```python
from build123d import *

# Parameters (mm, degrees)
F0_W     = 6.35
F0_H     = 88.9
F1_DEPTH = 3
F0_H_2   = 6.35
F0_W_2   = 12.7
F0_W_3   = 76.2
F2_DEPTH = 25.4
F0_W_4   = 25.4
F3_DEPTH = 8


with BuildPart() as f1:
    # F0 (on Front) → F1 (new body)
    with BuildSketch(Plane.XZ):
        with Locations((-59.3524831653, 10.6868692262)):
            Rectangle(F0_W, F0_H)
        Polygon((-43.4774831653, 55.1368692262), (-56.1774831653, 55.1368692262), (-56.1774831653, -33.7631307738), (-43.4774831653, -33.7631307738), (-18.0774831653, -33.7631307738), (58.1225168347, -33.7631307738), (83.5225168347, -33.7631307738), (96.2225168347, -33.7631307738), (96.2225168347, 55.1368692262), (83.5225168347, 55.1368692262), (58.1225168347, 55.1368692262), (-18.0774831653, 55.1368692262), align=None)
    extrude(amount=F1_DEPTH)

    # F0 (on Front) → F2 (join)
    with BuildSketch(Plane.XZ):
        with Locations((-59.3524831653, 58.3118692262)):
            Rectangle(F0_W, F0_H_2)
        with Locations((99.3975168347, 58.3118692262)):
            Rectangle(F0_W, F0_H_2)
        with Locations((-59.3524831653, -36.9381307738)):
            Rectangle(F0_W, F0_H_2)
        with Locations((99.3975168347, -36.9381307738)):
            Rectangle(F0_W, F0_H_2)
        with Locations((-49.8274831653, 58.3118692262)):
            Rectangle(F0_W_2, F0_H_2)
        with Locations((20.0225168347, 58.3118692262)):
            Rectangle(F0_W_3, F0_H_2)
        with Locations((89.8725168347, 58.3118692262)):
            Rectangle(F0_W_2, F0_H_2)
        with Locations((-49.8274831653, -36.9381307738)):
            Rectangle(F0_W_2, F0_H_2)
        with Locations((20.0225168347, -36.9381307738)):
            Rectangle(F0_W_3, F0_H_2)
        with Locations((89.8725168347, -36.9381307738)):
            Rectangle(F0_W_2, F0_H_2)
        with Locations((99.3975168347, 10.6868692262)):
            Rectangle(F0_W, F0_H)
        with Locations((-59.3524831653, 10.6868692262)):
            Rectangle(F0_W, F0_H)
    extrude(amount=F2_DEPTH)

    # F0 (on Front) → F3 (join)
    with BuildSketch(Plane.XZ):
        with Locations((-30.7774831653, -36.9381307738)):
            Rectangle(F0_W_4, F0_H_2)
        with Locations((-30.7774831653, 58.3118692262)):
            Rectangle(F0_W_4, F0_H_2)
        with Locations((70.8225168347, 58.3118692262)):
            Rectangle(F0_W_4, F0_H_2)
        with Locations((70.8225168347, -36.9381307738)):
            Rectangle(F0_W_4, F0_H_2)
    extrude(amount=F3_DEPTH)


solid = f1.part
```
The listing builds one solid part. Answer for the finished solid, in the listing's coordinates (mm). A direction names the side the tool comes from. Give positions to 0.01 mm unless a question says otherwise; leave off trailing zeros. Loops run counter-clockwise (first coordinate to the right, second up) from the corner with the lowest first, then second, coordinate; pieces in that order, holes last. Notation, with made-up numbers: (24.5, -12) - (70.5, -12) arc R5 cw to (70.5, -4) - close; hole circle Ø11 at (-23.5, -29). An arc over 180 degrees is marked (long way). Answer as CSV lines item,"result". Start each with the question number.
Item 1: A cutting plane is placed at A-A on y = -9.75. Determine the outline of the cut face in (x, z).
Item 2: A cutting plane is placed at B-B on x = 15. Determine the outline of the cut face in (y, z), then the cut area to 3 significant figures.
Item 3: Each of these flat-tipped pins is pushed along its axis until it touches: pin 1 (12 mm diameter, centred on x = 67, z = 15.5, fed in from +Y); pin 2 (7 mm diameter, centred on x = 71, z = -36, fed in from -Y); pin 3 (1.5 mm diameter, centred on x = 50, z = 51, fed in from -Y). Where does it stop, or does it pass through?
Item 4: The mould has two halves that part along X. Classify faces 4 (the face through (19, -14, -33.763)), 5 (the face through (19, -13, -40.113)), 6 (the face through (102.573, -13, 10)): +X half, -X half, draft (parallel to the pull), parting line (faces both ways), or undercut.
Item 5: A cutting plane is placed at C-C on z = 52. Determine the outline of the cut face in (x, y), then the cut area to 3 significant figures.
Item 6: For faces 1 (the face through (-18.077, -17, 58)), 2 (the face through (19, -14, 55.137)), 3 (the face through (21, -13, 61.487)), determine the directions among +Z, -Z, +X, -X, +Y, -Y from which every point of the face is accessible in a straight line to the end or side of a thin tool.
Item 7: Find the intervals of material crossed by line 1 (X direction, y = -16, z = -36); line 2 (Z direction, x = -23.5, y = -3.5); line 3 (X direction, y = -15.5, z = -30.5), in increasing order. Write a range as from..to.
Found:
1,outline,"(-62.53, -40.11) - (-43.48, -40.11) - (-43.48, -33.76) - (-56.18, -33.76) - (-56.18, 55.14) - (-43.48, 55.14) - (-43.48, 61.49) - (-62.53, 61.49) - close; (-18.08, -40.11) - (58.12, -40.11) - (58.12, -33.76) - (-18.08, -33.76) - close; (-18.08, 55.14) - (58.12, 55.14) - (58.12, 61.49) - (-18.08, 61.49) - close; (83.52, -40.11) - (102.57, -40.11) - (102.57, 61.49) - (83.52, 61.49) - (83.52, 55.14) - (96.22, 55.14) - (96.22, -33.76) - (83.52, -33.76) - close"
2,outline,"(-25.4, -40.11) - (0, -40.11) - (0, 61.49) - (-25.4, 61.49) - (-25.4, 55.14) - (-3, 55.14) - (-3, -33.76) - (-25.4, -33.76) - close"
2,area,"589 mm^2"
3,pin 1,"stops at y = 0"
3,pin 2,"stops at y = -8"
3,pin 3,"stops at y = -3"
4,face 4,"undercut"
4,face 5,"draft"
4,face 6,"+X half"
5,outline,"(-62.53, -25.4) - (-56.18, -25.4) - (-56.18, -3) - (96.22, -3) - (96.22, -25.4) - (102.57, -25.4) - (102.57, 0) - (-62.53, 0) - close"
5,area,"780 mm^2"
6,face 1,"+Z, -Z, -Y"
6,face 2,"-Y"
6,face 3,"+Z, +X, -X, +Y, -Y"
7,line 1,"x = -62.53..-43.48, -18.08..58.12, 83.52..102.57"
7,line 2,"z = -40.11..-33.76, 55.14..61.49"
7,line 3,"x = -62.53..-56.18, 96.22..102.57"
